Design review of the part built by this model. Coordinates are the model's own, in mm. Coordinates: 2 decimals unless noted, no trailing zeros. Write each loop counter-clockwise with the first axis right and the second up, starting at its lowest first coordinate (ties: lowest second). Pieces come first, ordered by that corner, then holes.
Q1. For probe 1 along X at (y, z) = (57.5, 0.35); probe 2 along X at (y, z) = (37, 0.95); probe 3 along Y at (x, z) = (-4, 2.05), list the stretches that pass through material, from the lowest coordinate up.
Q2. Take a section at B-B (z = 1). State how many separate pieces and enclosed holes the cut face has, and give its area (3 significant figures).
Q3. Take a section at C-C (y = 77). Give the boundary of the cut face in (x, z) (3 decimals).
Q4. Take a section at A-A (x = -14.5). Give the boundary of the cut face in (y, z) (3 decimals).
Q5. Insertion check: pin 1 (1 mm diameter, centred on x = -8.5, z = 1, fed in from +Y); pin 2 (1 mm diameter, centred on x = 8.5, z = 1.5, fed in from +Y); pin 3 (1.6 mm diameter, centred on x = 21, z = 1, fed in from +Y). Each pin has a flat end and moves straight along its axis. Give the tip position at first contact, or say it passes through.
Q6. Take a section at D-D (x = 42). Give the boundary of the cut face in (y, z) (3 decimals), and give its area (3 significant figures).
```python
from build123d import *

# Parameters (mm, degrees)
F1_DEPTH = 3.175


with BuildPart() as f1:
    # F0 (on Top) → F1 (new body)
    with BuildSketch(Plane.XY):
        with BuildLine():
            Line((-43.6475083196, 57.6062907483), (-43.6475083196, -69.3937092517))
            Line((-43.6475083196, -69.3937092517), (57.9524916804, -69.3937092517))
            Line((57.9524916804, -69.3937092517), (57.9524916804, 57.6062907483))
            Line((57.9524916804, 57.6062907483), (34.9589943423, 57.6062907483))
            add(Edge.make_bspline(
                [(34.9589943423, 57.6062907483), (38.056212694, 55.3623037103), (38.056212694, 50.7103741337)],
                knots=[0.4823776889, 0.4823776889, 0.4823776889, 1, 1, 1], degree=2))
            add(Edge.make_bspline(
                [(38.056212694, 50.7103741337), (38.056212694, 46.0243819592), (34.8590696182, 43.5024538941)],
                knots=[0, 0, 0, 1, 1, 1], degree=2))
            add(Edge.make_bspline(
                [(34.8590696182, 43.5024538941), (31.6619265424, 40.980525829), (25.7132822978, 40.980525829)],
                knots=[0, 0, 0, 1, 1, 1], degree=2))
            Line((25.7132822978, 40.980525829), (22.08062554, 40.980525829))
            Line((22.08062554, 40.980525829), (22.08062554, 28.846912086))
            Line((22.08062554, 28.846912086), (18.495233833, 28.846912086))
            Line((18.495233833, 28.846912086), (18.495233833, 57.6062907483))
            Line((18.495233833, 57.6062907483), (10.0347897484, 57.6062907483))
            Line((10.0347897484, 57.6062907483), (10.0347897484, 28.846912086))
            Line((10.0347897484, 28.846912086), (6.4493980414, 28.846912086))
            Line((6.4493980414, 28.846912086), (6.4493980414, 57.6062907483))
            Line((6.4493980414, 57.6062907483), (-3.5177150874, 57.6062907483))
            add(Edge.make_bspline(
                [(-3.5177150874, 57.6062907483), (-3.4643650115, 57.5651959541), (-3.4121171904, 57.5232935921)],
                knots=[0.9807273895, 0.9807273895, 0.9807273895, 1, 1, 1], degree=2))
            add(Edge.make_bspline(
                [(-3.4121171904, 57.5232935921), (-0.7011289223, 55.3491012575), (-0.7011289223, 50.980460138)],
                knots=[0, 0, 0, 1, 1, 1], degree=2))
            add(Edge.make_bspline(
                [(-0.7011289223, 50.980460138), (-0.7011289223, 44.8630121407), (-6.906354871, 42.7090762565)],
                knots=[0, 0, 0, 1, 1, 1], degree=2))
            Line((-6.906354871, 42.7090762565), (1.4730634123, 28.846912086))
            Line((1.4730634123, 28.846912086), (-2.7672868552, 28.846912086))
            Line((-2.7672868552, 28.846912086), (-10.2351648739, 41.67599729))
            Line((-10.2351648739, 41.67599729), (-16.6767160764, 41.67599729))
            Line((-16.6767160764, 41.67599729), (-16.6767160764, 28.846912086))
            Line((-16.6767160764, 28.846912086), (-20.2621077834, 28.846912086))
            Line((-20.2621077834, 28.846912086), (-20.2621077834, 57.6062907483))
            Line((-20.2621077834, 57.6062907483), (-43.6475083196, 57.6062907483))
        make_face()
        with BuildLine():
            ThreePointArc((57.9524916804, 57.6062907483), (7.1524916804, 108.4062907483), (-43.6475083196, 57.6062907483))
            Line((-43.6475083196, 57.6062907483), (-20.2621077834, 57.6062907483))
            Line((-20.2621077834, 57.6062907483), (-20.2621077834, 59.6974859266))
            Line((-20.2621077834, 59.6974859266), (-11.8016636989, 59.6974859266))
            add(Edge.make_bspline(
                [(-11.8016636989, 59.6974859266), (-6.2325460998, 59.6974859266), (-3.5177150874, 57.6062907483)],
                knots=[0, 0, 0, 0.9807273895, 0.9807273895, 0.9807273895], degree=2))
            Line((-3.5177150874, 57.6062907483), (6.4493980414, 57.6062907483))
            Line((6.4493980414, 57.6062907483), (6.4493980414, 59.6974859266))
            Line((6.4493980414, 59.6974859266), (10.0347897484, 59.6974859266))
            Line((10.0347897484, 59.6974859266), (10.0347897484, 57.6062907483))
            Line((10.0347897484, 57.6062907483), (18.495233833, 57.6062907483))
            Line((18.495233833, 57.6062907483), (18.495233833, 59.6974859266))
            Line((18.495233833, 59.6974859266), (26.4965317102, 59.6974859266))
            add(Edge.make_bspline(
                [(26.4965317102, 59.6974859266), (32.0726639073, 59.6974859266), (34.9589943423, 57.6062907483)],
                knots=[0, 0, 0, 0.4823776889, 0.4823776889, 0.4823776889], degree=2))
            Line((34.9589943423, 57.6062907483), (57.9524916804, 57.6062907483))
        make_face()
    extrude(amount=F1_DEPTH)


solid = f1.part
```
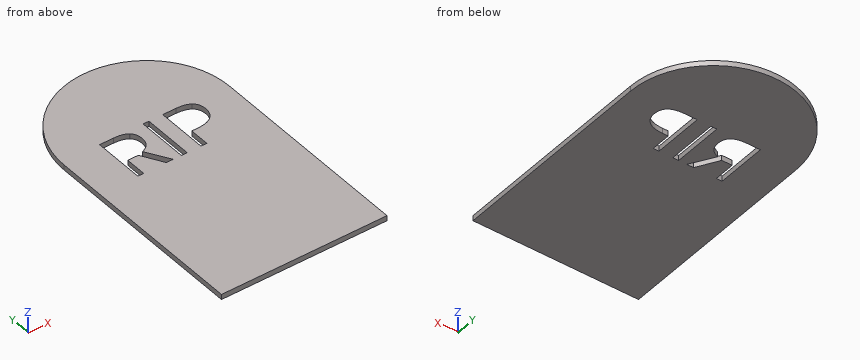
Response:
1. probe 1: x = -43.65 to -20.26, -3.38 to 6.45, 10.03 to 18.5, 35.1 to 57.95
1. probe 2: x = -43.65 to -20.26, -16.68 to -7.51, -3.46 to 6.45, 10.03 to 18.5, 22.08 to 57.95
1. probe 3: y = -69.39 to 30.96, 37.9 to 44.17, 57.95 to 107.17
2. separate pieces: 1
2. enclosed holes: 3
2. area: 16,100 mm2
3. outline: (-39.8, 0) - (54.105, 0) - (54.105, 3.175) - (-39.8, 3.175) - close
4. outline: (-69.394, 0) - (41.676, 0) - (41.676, 3.175) - (-69.394, 3.175) - close; (59.697, 0) - (103.561, 0) - (103.561, 3.175) - (59.697, 3.175) - close
5. pin 1: stops at y = 106.09
5. pin 2: stops at y = 108.4
5. pin 3: stops at y = 106.7
6. outline: (-69.394, 0) - (94.57, 0) - (94.57, 3.175) - (-69.394, 3.175) - close
6. area: 521 mm2
